Here's how the part is built. I have some questions about the finished solid (model axes, mm). A direction names the side the tool comes from. Give positions to 0.01 mm unless a question says otherwise; leave off trailing zeros.
from build123d import *

# Parameters (mm, degrees)
EXTRUDE_1_DEPTH          = 50
CUT_EXTRUDE_1_DEPTH      = 22
CUT_EXTRUDE_1_DEPTH_BACK = 22
CHAMFER_1_SIZE           = 10
CUT_EXTRUDE_4_DEPTH      = 38
SKETCH_7_R               = 2.7
CUT_EXTRUDE_5_DEPTH      = 158.237473694
SKETCH_12_W              = 10.5
SKETCH_12_H              = 10.5
CUT_EXTRUDE_8_DEPTH      = 4
SKETCH_13_W              = 10
SKETCH_13_H              = 10
EXTRUDE_3_DEPTH          = 3.5
EXTRUDE_4_DEPTH          = 6
SKETCH_16_R              = 10.05
CUT_EXTRUDE_11_DEPTH     = 3
SKETCH_17_R              = 4.5
CUT_EXTRUDE_12_DEPTH     = 158.41319251
SKETCH_18_R              = 30
CUT_EXTRUDE_13_DEPTH     = 6
FILLET_1_2_ANGLE         = 72
FILLET_1_3_ANGLE         = 72
FILLET_1_4_ANGLE         = 72


with BuildPart() as part:
    # 草图1 → 凸台-拉伸1 (new body)
    with BuildSketch(Plane.XY):
        with BuildLine():
            Line((0, 0), (0, 110))
            ThreePointArc((0, 110), (64.656377752, 88.991869381), (104.616216792, 33.991869381))
            Line((104.616216792, 33.991869381), (0, 0))
        make_face()
    extrude(amount=EXTRUDE_1_DEPTH)

    # 草图2 → 切除-拉伸1 (cut, two sides: drawn at the far end of the back side and taken through both)
    with BuildSketch(Plane(origin=(0, 0, 0), x_dir=(0, 0, 1), z_dir=(-0.8090169943749467, 0.5877852522924744, 0)).offset(-CUT_EXTRUDE_1_DEPTH_BACK)):
        with BuildLine():
            Line((-2.434479972, 121.031505263), (-32.434479972, 60.021300119))
            ThreePointArc((-32.434479972, 60.021300119), (-25.826576487, 29.63728916), (5.26447133, 29.190908144))
            ThreePointArc((5.26447133, 29.190908144), (34.528838333, 64.97494707), (45, 110))
            ThreePointArc((45, 110), (25.662949792, 134.35017453), (-2.434479972, 121.031505263))
        make_face()
    extrude(amount=CUT_EXTRUDE_1_DEPTH + CUT_EXTRUDE_1_DEPTH_BACK, mode=Mode.SUBTRACT)

    # 倒角1
    # the kernel refuses this chamfer: 10 mm, written as the material it takes off along each edge
    with BuildSketch(Plane(origin=(-15.115973339, 16.623283153, 0), x_dir=(0, 0, 1), z_dir=(0.5877852522924744, 0.8090169943749467, 0))) as chamfer_1_piece_1_section:
        Polygon((CHAMFER_1_SIZE, 0), (0, -CHAMFER_1_SIZE), (0, 0), align=None)
    chamfer_1_piece_1 = extrude(amount=128.930806191, mode=Mode.PRIVATE)
    chamfer_1_piece_1 = chamfer_1_piece_1 & Plane(origin=(46.858003876, 101.923144932, -57.037418863), x_dir=(-0.4654997448337989, -0.6407054327731835, 0.6105788531996469), z_dir=(0.8090169943749466, -0.5877852522924744, 0)) * Cylinder(102.037418863, 298, mode=Mode.PRIVATE)
    add(chamfer_1_piece_1, mode=Mode.SUBTRACT)
    with BuildSketch(Plane(origin=(20.480774414, -9.239267947, 0), x_dir=(0, 0, 1), z_dir=(0.5877852522924744, 0.8090169943749467, 0))) as chamfer_1_piece_2_section:
        Polygon((CHAMFER_1_SIZE, 0), (0, CHAMFER_1_SIZE), (0, 0), align=None)
    chamfer_1_piece_2 = extrude(amount=128.930806191, mode=Mode.PRIVATE)
    chamfer_1_piece_2 = chamfer_1_piece_2 & Plane(origin=(82.454751628, 76.060593831, -57.037418863), x_dir=(-0.4654997448337989, -0.6407054327731835, 0.6105788531996469), z_dir=(0.8090169943749466, -0.5877852522924744, 0)) * Cylinder(102.037418863, 298, mode=Mode.PRIVATE)
    add(chamfer_1_piece_2, mode=Mode.SUBTRACT)

    # 草图5 → 切除-旋转2 (revolve, cut)
    with BuildSketch(Plane(origin=(0, 0, 0), x_dir=(0, 0, 1), z_dir=(-0.8090169943749467, 0.5877852522924744, 0))):
        with BuildLine():
            Line((38.64565174, 61), (38.64565174, 0))
            Line((38.64565174, 0), (50.462581137, 0))
            Line((50.462581137, 0), (50.462581137, 110))
            ThreePointArc((50.462581137, 110), (47.466600414, 84.797620051), (38.64565174, 61))
        make_face()
        with BuildLine():
            Line((-5, 24), (-5, 0))
            Line((-5, 0), (33.64565174, 0))
            Line((33.64565174, 0), (33.64565174, 52.269326125))
            ThreePointArc((33.64565174, 52.269326125), (21.831047905, 36.951968201), (7.462581137, 24))
            Line((7.462581137, 24), (-5, 24))
        make_face()
    revolve(axis=Axis((0, 0, -7.898129057), (0, 0, 1)), mode=Mode.SUBTRACT)

    # 草图6 → 切除-拉伸4 (cut)
    with BuildSketch(Plane(origin=(0, 0, 0), x_dir=(-1, 0, 0), z_dir=(0, 0, -1))):
        Polygon((-4, 59.947179416), (-4, 121.087474703), (-38.681182805, 107.68173241), align=None)
        Polygon((-90.458270445, 70.063476264), (-113.924963881, 41.222313554), (-55.77708764, 22.32892327), align=None)
    extrude(amount=-CUT_EXTRUDE_4_DEPTH, mode=Mode.SUBTRACT)

    # 草图7 → 切除-拉伸5 (cut, through all)
    with BuildSketch(Plane(origin=(4, 0, 0), x_dir=(0, 0, -1), z_dir=(1, 0, 0))):
        with Locations((-20, 99.927248669)):
            Circle(SKETCH_7_R)
        with Locations((-20, 74.927248669)):
            Circle(SKETCH_7_R)
    cut_extrude_5 = extrude(amount=-CUT_EXTRUDE_5_DEPTH, mode=Mode.SUBTRACT)

    # 镜向1: 切除-拉伸5 across plane
    add(cut_extrude_5.mirror(Plane(origin=(0, 0, 0), x_dir=(0, 0, 1), z_dir=(-0.8090169943749466, 0.5877852522924742, 0))), mode=Mode.SUBTRACT)

    # 草图12 → 切除-拉伸8 (cut)
    with BuildSketch(Plane.ZY):
        with Locations((20, 55)):
            Rectangle(SKETCH_12_W, SKETCH_12_H)
    extrude(amount=-CUT_EXTRUDE_8_DEPTH, mode=Mode.SUBTRACT)

    # 草图13 → 凸台-拉伸3 (add)
    with BuildSketch(Plane(origin=(0, 0, 0), x_dir=(0.9510565162951544, 0.30901699437494484, 0), z_dir=(0.30901699437494484, -0.9510565162951544, 0))):
        with Locations((55, 20)):
            Rectangle(SKETCH_13_W, SKETCH_13_H)
    extrude(amount=EXTRUDE_3_DEPTH)

    # 草图14 → 凸台-拉伸4 (add)
    with BuildSketch(Plane.XY.offset(38.64565174)):
        with BuildLine():
            Line((0, 0), (0, 40))
            ThreePointArc((0, 40), (23.511410092, 32.360679775), (38.042260652, 12.360679775))
            Line((38.042260652, 12.360679775), (0, 0))
        make_face()
    extrude(amount=EXTRUDE_4_DEPTH)

    # 草图16 → 切除-拉伸11 (cut)
    with BuildSketch(Plane.XY.offset(44.64565174)):
        Circle(SKETCH_16_R)
    extrude(amount=-CUT_EXTRUDE_11_DEPTH, mode=Mode.SUBTRACT)

    # 草图17 → 切除-拉伸12 (cut, through all)
    with BuildSketch(Plane.XY.offset(41.64565174)):
        Circle(SKETCH_17_R)
    extrude(amount=-CUT_EXTRUDE_12_DEPTH, mode=Mode.SUBTRACT)

    # 草图18 → 切除-拉伸13 (cut)
    with BuildSketch(Plane(origin=(0, 0, 33.64565174), x_dir=(-1, 0, 0), z_dir=(0, 0, -1))):
        Circle(SKETCH_18_R)
    extrude(amount=-CUT_EXTRUDE_13_DEPTH, mode=Mode.SUBTRACT)

    # 圆角1: read off the stored shape, not the designer's step
    # 圆角1 outline → 圆角1 (revolve, cut)
    with BuildSketch(Plane.XZ):
        with BuildLine():
            ThreePointArc((30, 36.64565174), (29.802517077, 37.716118009), (29.236067978, 38.64565174))
            Line((29.236067978, 38.64565174), (27, 38.64565174))
            Line((27, 38.64565174), (27, 33.64565174))
            Line((27, 33.64565174), (33, 33.64565174))
            ThreePointArc((33, 33.64565174), (30.878679657, 34.524331396), (30, 36.64565174))
        make_face()
    revolve(axis=Axis((0, 0, 0), (0, 0, 1)), mode=Mode.SUBTRACT)

    # Fillet 1 2 outline → Fillet 1 2 (revolve)
    with BuildSketch(Plane(origin=(0, 0, 0), x_dir=(0.9510565162951545, 0.30901699437494434, 0), z_dir=(0.30901699437494434, -0.9510565162951545, 0))):
        with BuildLine():
            Line((30, 39.64565174), (27, 39.64565174))
            ThreePointArc((27, 39.64565174), (29.121320344, 38.766972084), (30, 36.64565174))
            Line((30, 36.64565174), (30, 39.64565174))
        make_face()
    revolve(axis=Axis((0, 0, 0), (0, 0, 1)), revolution_arc=FILLET_1_2_ANGLE)

    # Fillet 1 3 outline → Fillet 1 3 (revolve)
    with BuildSketch(Plane(origin=(0, 0, 0), x_dir=(0.9510565162951548, 0.30901699437494395, 0), z_dir=(0.30901699437494395, -0.9510565162951548, 0))):
        with BuildLine():
            ThreePointArc((43, 38.64565174), (40.878679657, 39.524331397), (40, 41.64565174))
            ThreePointArc((40, 41.64565174), (39.121320344, 43.766972084), (37, 44.64565174))
            Line((37, 44.64565174), (37, 38.64565174))
            Line((37, 38.64565174), (43, 38.64565174))
        make_face()
    revolve(axis=Axis((0, 0, 0), (0, 0, 1)), revolution_arc=FILLET_1_3_ANGLE)

    # Fillet 1 4 outline → Fillet 1 4 (revolve, cut)
    with BuildSketch(Plane(origin=(0, 0, 0), x_dir=(0.9510565162951548, 0.30901699437494395, 0), z_dir=(0.30901699437494395, -0.9510565162951548, 0))):
        with BuildLine():
            ThreePointArc((37, 44.64565174), (39.121320344, 43.766972084), (40, 41.64565174))
            ThreePointArc((40, 41.64565174), (40.878679657, 39.524331397), (43, 38.64565174))
            Line((43, 38.64565174), (43, 44.64565174))
            Line((43, 44.64565174), (37, 44.64565174))
        make_face()
    revolve(axis=Axis((0, 0, 0), (0, 0, 1)), revolution_arc=FILLET_1_4_ANGLE, mode=Mode.SUBTRACT)


solid = part.part
Q1. For faces 1 (the face through (4, 55, 20)), 2 (the face through (14.28, 19.29, 3.68)), 3 (the face through (14, 20, 44.646)), which set-ups out of +Z, -Z, +X, -X, +Y, -Y let a thin tool reach every point of the face, with its end or its side?
Filled sheet:
face 1: -X
face 2: -Z, -X, -Y
face 3: +Z, -X, -Y
Q2. I need wall thicknesses on L1, parallel to Y at x = 2.8, z = 20; L2, parallel to X at y = 61, z = 9; L3, parallel to X at y = 70.5, z = 17.5. Which ranges of each line are inside material? Lowest first, please.
Filled sheet:
L1: y = 34.91 to 49.75, 60.25 to 72.23, 77.63 to 97.23, 102.63 to 109.96
L2: x = 0 to 4, 4.76 to 15.89, 72.75 to 83.87
L3: x = 0 to 4, 11.67 to 24.03, 78.41 to 84.44
Q3. I'm going to push flat-ended pins straight in: P1, Ø4.5, axis at x = 4.5, y = 7, coming from the +Z side; P2, Ø5, axis at x = 17.5, z = 10, coming from the -Y side; P3, Ø3, axis at y = 53.5, z = 21, coming from the -X side. Where does each tip first touch, or does it pass through?
Filled sheet:
P1: stops at z = 44.65
P2: stops at y = 15.27
P3: stops at x = 4
Q4. If we section it at A-A on z = 20: Give the number of separate pieces and of enclosed holes in the cut face, plus the area to 3 significant figures.
Filled sheet:
separate pieces: 6
enclosed holes: 0
area: 2,180 mm2
Q5. Thinking about a two-plate mould opening in Y: for faces 4 (the face through (20.21, 82.26, 18.73)), 5 (the face through (69.65, 24.763, 17.506)), 6 (the face through (60, 82, 50)), which applies, released by +Y, released by -Y, zero draft, split by the parting line, or undercut?
Filled sheet:
face 4: released by +Y
face 5: undercut
face 6: zero draft
